```python
from build123d import *

# Parameters (mm, degrees)
ESBO_O1_R                = 3.75
RESSALTO_EXTRUS_O1_DEPTH = 50
RESSALTO_EXTRUS_O2_DEPTH = 2
ESBO_O3_W                = 3
ESBO_O3_H                = 10
RESSALTO_EXTRUS_O3_DEPTH = 42.2
ESBO_O4_W                = 2
ESBO_O4_H                = 10
RESSALTO_EXTRUS_O4_DEPTH = 5
ESBO_O5_W                = 2
ESBO_O5_H                = 10
RESSALTO_EXTRUS_O5_DEPTH = 5
FILETE1_R                = 1.5
ESBO_O6_R                = 1.5
CORTE_EXTRUS_O1_DEPTH    = 5


with BuildPart() as part:
    # Esboço1 → Ressalto-extrusão1 (new body)
    with BuildSketch(Plane.XY):
        Circle(ESBO_O1_R)
    extrude(amount=RESSALTO_EXTRUS_O1_DEPTH)

    # Esboço2 → Ressalto-extrusão2 (add)
    with BuildSketch(Plane.XY.offset(50)):
        with BuildLine():
            Line((0, 5), (0, 3.75))
            ThreePointArc((0, 3.75), (2.651650429, 2.651650429), (3.75, 0))
            ThreePointArc((3.75, 0), (2.651650429, -2.651650429), (0, -3.75))
            Line((0, -3.75), (0, -5))
            Line((0, -5), (25, -5))
            Line((25, -5), (25, 5))
            Line((25, 5), (0, 5))
        make_face()
        with BuildLine():
            ThreePointArc((0, -3.75), (-3.75, 0), (0, 3.75))
            Line((0, 3.75), (0, 5))
            Line((0, 5), (-25, 5))
            Line((-25, 5), (-25, -5))
            Line((-25, -5), (0, -5))
            Line((0, -5), (0, -3.75))
        make_face()
        with BuildLine():
            Line((0, -3.75), (0, 0))
            Line((0, 0), (0, 3.75))
            ThreePointArc((0, 3.75), (-3.75, 0), (0, -3.75))
        make_face()
        with BuildLine():
            Line((0, 3.75), (0, 0))
            Line((0, 0), (0, -3.75))
            ThreePointArc((0, -3.75), (2.651650429, -2.651650429), (3.75, 0))
            ThreePointArc((3.75, 0), (2.651650429, 2.651650429), (0, 3.75))
        make_face()
    extrude(amount=RESSALTO_EXTRUS_O2_DEPTH)

    # Esboço3 → Ressalto-extrusão3 (add)
    with BuildSketch(Plane.XY.offset(52)):
        with Locations((-23.5, 0)):
            Rectangle(ESBO_O3_W, ESBO_O3_H)
        with Locations((23.5, 0)):
            Rectangle(ESBO_O3_W, ESBO_O3_H)
    extrude(amount=RESSALTO_EXTRUS_O3_DEPTH)

    # Esboço4 → Ressalto-extrusão4 (add)
    with BuildSketch(Plane(origin=(-22, 0, 0), x_dir=(0, 0, -1), z_dir=(1, 0, 0))):
        with Locations((-93.2, 0)):
            Rectangle(ESBO_O4_W, ESBO_O4_H)
    extrude(amount=RESSALTO_EXTRUS_O4_DEPTH)

    # Esboço5 → Ressalto-extrusão5 (add)
    with BuildSketch(Plane.ZY.offset(-22)):
        with Locations((93.2, 0)):
            Rectangle(ESBO_O5_W, ESBO_O5_H)
    extrude(amount=RESSALTO_EXTRUS_O5_DEPTH)

    # Filete1
    filete1_edges = [part.edges().sort_by_distance(p)[0] for p in [
        (-3.75, 0, 50),
    ]]
    fillet(filete1_edges, radius=FILETE1_R)

    # Esboço6 → Corte-extrusão1 (cut, symmetric)
    with BuildSketch(Plane(origin=(0, 0, 0), x_dir=(1, 0, 0), z_dir=(0, 1, 0))):
        with Locations(Location((0, -45, 0), (0, 0, 270))):
            Circle(ESBO_O6_R)
    extrude(amount=CORTE_EXTRUS_O1_DEPTH, both=True, mode=Mode.SUBTRACT)


solid = part.part
```
Build history of the part. All positions in model axes, mm. A direction names the side the tool comes from. Coordinates: 2 decimals unless noted, no trailing zeros. Order: outer loops, then holes, each group sorted by start corner. A loop starts at its lowest first (then second) coordinate and runs counter-clockwise, first axis right, second up. Notation, with made-up numbers: M 71.5,60.25 L 102.5,60.25 A28 cw 102.5,79.25 Z; hole C -33,57 d2. An arc over 180 degrees is marked long. One line per question, with ' | ' between items. Start each with the question number.
1. Tool access for faces 1 (the face through (20, 0, 92.2)), 2 (the face through (-21, 0, 94.2)), 3 (the face through (-17, 0, 93)), 4 (the face through (3.577, 1.126, 23.926)), 5 (the face through (0, -5, 51)): list every direction of +Z, -Z, +X, -X, +Y, -Y with a clear straight run to the whole face (end or side of a thin tool).
2. Cut at A-A (z = 76). Write the cut outline in (x, y).
3. Wall check: line 1 along Z through (x, y) = (0, 0.25); line 2 along X through (y, z) = (-1.5, 72); line 3 along Z through (x, y) = (20, 4.25). Give the ranges that are in metal, low to high. Write a range as [from, to].
4. Flat gauge pins, fed straight in: P1, Ø2.5, axis at x = -18.5, y = 1.5, coming from the -Z side; P2, Ø3, axis at x = -6, y = 0, coming from the +Z side. Where does each tip first touch, or does it go through?
5. Cut at C-C (y = 0). Write the cut outline in (x, z), plus the area to 3 significant figures.
6. Mould opens along Z. For faces 6 (the face through (-22, 0, 72)), 7 (the face through (21, 0, 94.2)), 8 (the face through (17, 0, 93)) say: +Z half, -Z half, draft (parallel to the pull), parting line (faces both ways), or undercut.
7. Cut at B-B (x = 20.5). Write the cut outline in (y, z), plus the area to 3 significant figures.
8. Cut at D-D (z = 35). Write the cut outline in (x, y), plus the area to 3 significant figures.
The answers:
1) face 1: +Y, -Y | face 2: +Z, +X, -X, +Y, -Y | face 3: +Z, +Y, -Y | face 4: -Z | face 5: +Z, -Z, +X, -X, -Y
2) outline: M -25,-5 L -22,-5 L -22,5 L -25,5 Z; M 22,-5 L 25,-5 L 25,5 L 22,5 Z
3) line 1: z = [0, 43.5], [46.5, 52] | line 2: x = [-25, -22], [22, 25] | line 3: z = [50, 52], [92.2, 94.2]
4) P1: stops at z = 50 | P2: stops at z = 52
5) outline: M -25,50 L -5.25,50 A1.5 cw -3.75,48.5 L -3.75,0 L 3.75,0 L 3.75,48.5 A1.5 cw 5.25,50 L 25,50 L 25,94.2 L 17,94.2 L 17,92.2 L 22,92.2 L 22,52 L -22,52 L -22,92.2 L -17,92.2 L -17,94.2 L -25,94.2 Z; hole C 0,45 d3 | area: 742 mm2
6) face 6: undercut | face 7: +Z half | face 8: draft
7) outline: M -5,50 L 5,50 L 5,52 L -5,52 Z; M -5,92.2 L 5,92.2 L 5,94.2 L -5,94.2 Z | area: 40.0 mm2
8) outline: C 0,0 d7.5 | area: 44.2 mm2
